Here's the drawing with two shaded views (mm, measured from the low corner). I have some questions. A direction names the side the tool comes from. Round coordinates to 2 decimals unless told otherwise and drop trailing zeros. Write each loop counter-clockwise with the first axis right and the second up, starting at its lowest first coordinate (ties: lowest second). Pieces come first, ordered by that corner, then holes. Notation, with made-up numbers: M 3.25,88 L 57.25,88 A14 ccw 57.25,97 Z; hole C 48,-28.5 d11. An arc over 180 degrees is marked long. Write item = value, one per line. Start each with the question number.
(1) I want a section at B-B (z = 6). List the corners of the cut face in (x, y) for me, and give its area (3 significant figures).
(2) I need wall thicknesses on line 1 along X through (y, z) = (30, 4.25); line 2 along X through (y, z) = (28, 12.25) (1 decimal); line 3 along Z through (x, y) = (2, 23). Which ranges of each line are inside material? Lowest first, please.
(3) I want a section at A-A (y = 30). List the corners of the cut face in (x, z) for me.
(4) I want a section at C-C (y = 55.5). List the corners of the cut face in (x, z) for me.
(5) If we mould it in two halves opening along X, with no side actions, what happens to the marked faces 3, 4 and 5? For each: released by +X, released by -X, zero draft, split by the parting line, or undercut.
(6) Will these pins go through, and if not, where does the flat tip stop? pin 1 Ø10.5 at (x, y) = (27, 30) entering from -Z; pin 2 Ø5.5 at (x, y) = (26, 29) entering from +Z; pin 3 Ø10 at (y, z) = (44.5, 12.5) entering from -X (1 decimal); pin 4 Ø1.5 at (x, z) = (7.5, 5) entering from -Y.
(7) On a 3-axis mill with a long thin cutter (end or side, diameter ignored), from which of +Z, -Z, +X, -X, +Y, -Y can I reach the whole of each face in a straight line? I mean the marked faces 1 and 2. Say none if no direction works.
(8) I want a section at D-D (y = 7.5). List the corners of the cut face in (x, z) for me, and give its area (3 significant figures).
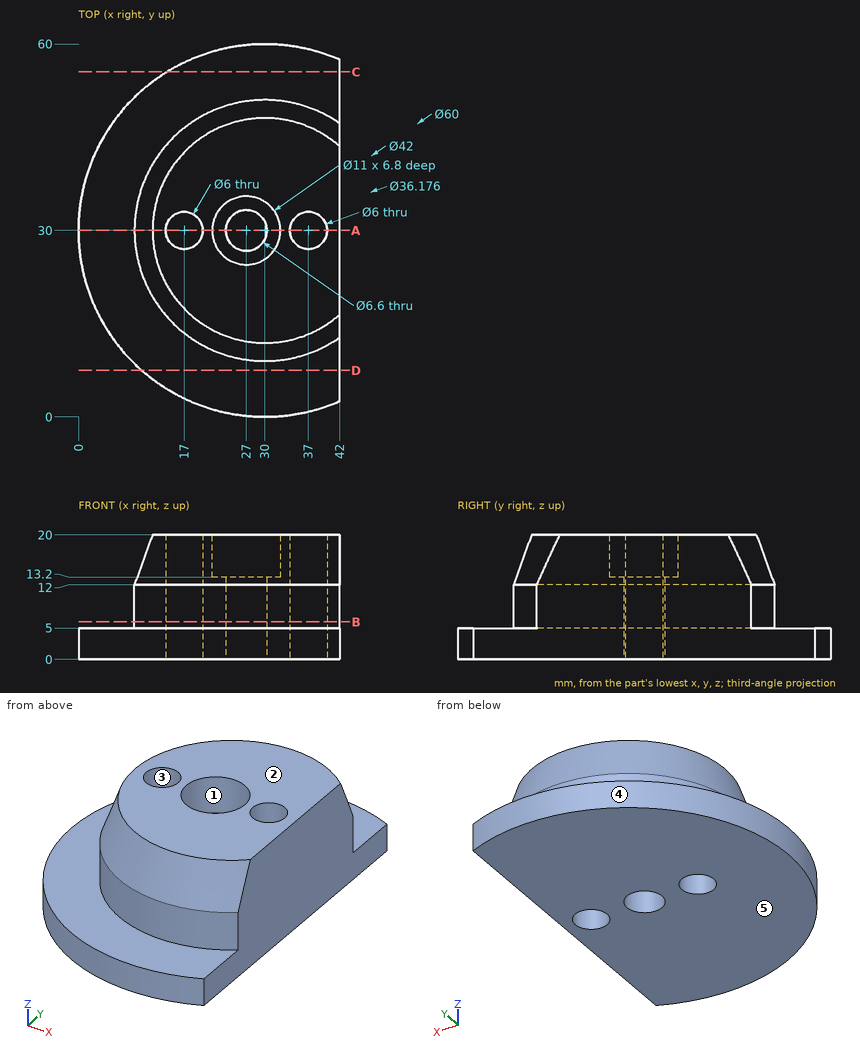
Returned:
q1.outline = M 42,12.77 L 42,47.23 A21 ccw long Z; hole C 17,30 d6; hole C 27,30 d6.6; hole C 37,30 d6
q1.area = 1,080 mm²
q2.line_1 = 0 to 14, 20 to 23.7, 30.3 to 34, 40 to 42
q2.line_2 = 9.2 to 14.8, 19.2 to 24.4, 29.6 to 34.8, 39.2 to 42
q2.line_3 = 0 to 5
q3.outline = M 0,0 L 14,0 L 14,20 L 11.91,20 L 9,12 L 9,5 L 0,5 Z; M 20,0 L 23.7,0 L 23.7,13.2 L 21.5,13.2 L 21.5,20 L 20,20 Z; M 30.3,0 L 34,0 L 34,20 L 32.5,20 L 32.5,13.2 L 30.3,13.2 Z; M 40,0 L 42,0 L 42,20 L 40,20 Z
q4.outline = M 14.2,0 L 42,0 L 42,5 L 14.2,5 Z
q5.face_3 = undercut
q5.face_4 = split by the parting line
q5.face_5 = zero draft
q6.pin_1 = 0
q6.pin_2 = 13.2
q6.pin_3 = 11.3
q6.pin_4 = 9.34
q7.face_1 = +Z
q7.face_2 = +Z, +X, -X, +Y, -Y
q8.outline = M 10.16,0 L 42,0 L 42,5 L 10.16,5 Z
q8.area = 159 mm²
